Source: CAD feature listing. Evaluate the final solid. Frame: model axes, mm. A direction names the side the tool comes from. Coordinates: 2 decimals unless noted, no trailing zeros. Loops run counter-clockwise (first coordinate to the right, second up) from the corner with the lowest first, then second, coordinate; pieces in that order, holes last.
Autodesk Inventor part; units mm, degrees
ref_plane "YZ Plane" through (0, 0, 0) normal (1, 0, 0) x (0, 1, 0)
ref_plane "XZ Plane" through (0, 0, 0) normal (0, 1, 0) x (-1, 0, 0)
ref_plane "XY Plane" through (0, 0, 0) normal (0, 0, 1) x (1, 0, 0)
sketch "Sketch1" plane through (0, 0, 0) normal (0, 0, 1) x (1, 0, 0)
  line L0 (0, 0) -> (406.4, 0)
  line L1 (406.4, 0) -> (406.4, 203.2)
  line L2 (406.4, 203.2) -> (0, 203.2)
  line L3 (0, 203.2) -> (0, 0)
  line L4 (0, 101.6) -> (664.7751, 101.6)
  line L5 (101.6, 101.6) -> (406.4, 50.8)
  line L6 (0, 50.8) -> (101.6, 50.8)
  line L7 (101.6, 50.8) -> (101.6, 0)
  line L8 (101.6, 101.6) -> (101.6, 203.2)
  arc A0 (101.6, 203.2) -> (233.5206, 79.6132) centre (256.07, 235.8848) ccw
  point P0 (226.7178, 80.747)
  dimension "d0" = 406.4
  dimension "d1" = 203.2
  dimension "d2" = 101.6
  dimension "d3" = 50.8
  dimension "d26" = 101.6
extrude "Extrusion1" add sketch "Sketch1" along normal blind 101.6 contours L7 L6 L3 L4 L5 A0 L1 L0 | L8 A0 L4 | L4 A0 L5 | A0 L5
chamfer "Chamfer1" distance 25.4 angle 45 1 edges at (406.4, 50.8, 50.8)
sketch "Sketch2" plane through (0, 50.8, 0) normal (0, -1, 0) x (1, 0, 0)
  circle A0 centre (25.4, 76.2) radius 3.175
  circle A1 centre (76.2, 76.2) radius 3.175
  circle A2 centre (76.2, 25.4) radius 3.175
  circle A3 centre (50.8, 50.8) radius 3.175
  circle A4 centre (25.4, 25.4) radius 3.175
  line L0 (0, 101.6) -> (101.6, 101.6)
  line L1 (0, 0) -> (0, 101.6)
  line L2 (101.6, 0) -> (101.6, 101.6)
  line L3 (0, 0) -> (101.6, 0)
  dimension "d9" = 6.35
  dimension "d10" = 6.35
  dimension "d11" = 6.35
  dimension "d12" = 6.35
  dimension "d13" = 6.35
  dimension "d14" = 25.4
  dimension "d15" = 25.4
  dimension "d16" = 25.4
  dimension "d17" = 25.4
  dimension "d18" = 25.4
  dimension "d19" = 25.4
  dimension "d20" = 25.4
  dimension "d21" = 25.4
  dimension "d22" = 50.8
  dimension "d23" = 50.8
extrude "Extrusion2" cut sketch "Sketch2" against normal blind 101.6 contours A0 | A1 | A2 | A3 | A4
properties part number "Table foot X4"
Q1. Contact query for flat-ended pins moving along their axis: pin 1 Ø4 at (y, z) = (172, 89) entering from +X; pin 2 Ø4 at (x, z) = (76.2, 25.4) entering from +Y; pin 3 Ø4 at (x, z) = (90.5, 25.5) entering from +Y; pin 4 Ø8 at (x, z) = (76.5, 84.5) entering from -Y. Output: stop coordinate, or through.
Q2. Line query: line 1 along Z through (x, y) = (25, 87); line 2 along Z through (x, y) = (25.4, 85) (3 decimals); line 3 along Y through (x, z) = (30.5, 20). Output: solid intervals per line, ascending.
Q3. Section B-B, the plane y = 95. Return the cut outline in (x, z) (3 decimals), plus the area to 3 significant figures.
Q4. Section A-A, the plane z = 84. Return the cut outline in (x, y).
Q5. Section C-C, the plane x = 269. Return the cut outline in (y, z), plus the area to 3 significant figures.
Q6. Access query for faces 1 (the flat face through (101.6, 26, 50)), 2 (the flat face through (101.6, 152, 50)), 3 (the cylindrical face through (146.565, 122.14, 50.089)). Directions: +Z, -Z, +X, -X, +Y, -Y. A direction counts if a zero-diameter tool reaches every point of the face in a straight line with its end or side. Return the directions, or none.
Q7. Section D-D, the plane y = 187.5. Return the cut outline in (x, z).
Derived:
1. pin 1: stops at x = 112.58
1. pin 2: passes through
1. pin 3: stops at y = 101.6
1. pin 4: stops at y = 50.8
2. line 1: z = 0 to 22.25, 28.55 to 73.05, 79.35 to 101.6
2. line 2: z = 0 to 22.225, 28.575 to 73.025, 79.375 to 101.6
2. line 3: y = 50.8 to 101.6
3. outline: (0, 0) - (184.791, 0) - (184.791, 101.6) - (0, 101.6) - close; hole circle Ø6.35 at (25.4, 25.4); hole circle Ø6.35 at (25.4, 76.2); hole circle Ø6.35 at (50.8, 50.8); hole circle Ø6.35 at (76.2, 25.4); hole circle Ø6.35 at (76.2, 76.2)
3. area: 18,600 mm2
4. outline: (0, 50.8) - (101.6, 50.8) - (101.6, 0) - (406.4, 0) - (406.4, 25.4) - (381.35, 54.98) - (226.72, 80.75) arc R157.89 cw to (101.6, 203.2) - (101.6, 101.6) - (0, 101.6) - close
5. outline: (0, 0) - (73.7, 0) - (73.7, 101.6) - (0, 101.6) - close
5. area: 7,490 mm2
6. face 1: +Z, -Z, -X, -Y
6. face 2: +Z, -Z, -X, +Y
6. face 3: +Z, -Z, +X, +Y
7. outline: (101.6, 0) - (105.78, 0) - (105.78, 101.6) - (101.6, 101.6) - close
